Part model, mm, in its own coordinate system. A direction names the side the tool comes from. Round coordinates to 2 decimals unless told otherwise and drop trailing zeros. Write each loop counter-clockwise with the first axis right and the second up, starting at its lowest first coordinate (ties: lowest second). Pieces come first, ordered by that corner, then holes.
```python
from build123d import *

# Parameters (mm, degrees)
EXTRUDE_1_DEPTH     = 10
FILLET_1_R          = 2
CUT_EXTRUDE_1_DEPTH = 11
CUT_EXTRUDE_2_DEPTH = 11


with BuildPart() as part:
    # 草图1 → 凸台-拉伸1 (new body)
    with BuildSketch(Plane.XY):
        Polygon((-26.953865184, 1.151568381), (-21.953865184, 1.151568381), (-21.953865184, 11.151568381), (11.796134816, 11.151568381), (11.796134816, 1.151568381), (16.796134816, 1.151568381), (16.796134816, 16.151568381), (-26.953865184, 16.151568381), align=None)
    extrude(amount=EXTRUDE_1_DEPTH)

    # 圆角1
    fillet_1_edges = [part.edges().sort_by_distance(p)[0] for p in [
        (-26.953865184, 16.151568381, 5),
        (16.796134816, 16.151568381, 5),
    ]]
    fillet(fillet_1_edges, radius=FILLET_1_R)

    # 草图2 → 切除-拉伸1 (cut, through all)
    with BuildSketch(Plane.XY.offset(10)):
        Polygon((-26.953865184, 1.151568381), (-21.953865184, 1.151568381), (-26.953865184, 5.718181818), align=None)
    extrude(amount=-CUT_EXTRUDE_1_DEPTH, mode=Mode.SUBTRACT)

    # 草图3 → 切除-拉伸2 (cut, through all)
    with BuildSketch(Plane.XY.offset(10)):
        Polygon((16.796134816, 5.718181818), (11.796134816, 1.151568381), (16.796134816, 1.151568381), align=None)
    extrude(amount=-CUT_EXTRUDE_2_DEPTH, mode=Mode.SUBTRACT)


solid = part.part
```
Q1. Cut at C-C on x = -1. Write the cut outline in (y, z).
Values follow:
outline: (11.15, 0) - (16.15, 0) - (16.15, 10) - (11.15, 10) - close
Q2. Which spindle directions (+Z, -Z, +X, -X, +Y, -Y) get a long thin tool onto all of the face, cutting with end or side? Do faces 4 (the flat face through (11.796, 6, 5)), 5 (the cylindrical face through (16.226, 15.55, 5.07)). Say none if no direction does.
Values follow:
face 4: +Z, -Z, -Y
face 5: +Z, -Z, +X, +Y
Q3. Wall check: L1, parallel to X at y = 9.25, z = 6; L2, parallel to Y at x = -9.5, z = 0.75; L3, parallel to X at y = 4.75, z = 2.25. Give the ranges that are in metal, low to high.
Values follow:
L1: x = -26.95 to -21.95, 11.8 to 16.8
L2: y = 11.15 to 16.15
L3: x = -25.89 to -21.95, 11.8 to 15.74
Q4. Drop flat-ended pins along their axis: pin 1 (3 mm diameter, centred on x = 6, z = 5.5, fed in from -Y); pin 2 (4 mm diameter, centred on x = -21, y = 10, fed in from -Z). Give the stop position or say it passes through.
Values follow:
pin 1: stops at y = 11.15
pin 2: stops at z = 0
Q5. Cut at A-A on y = 9.5. Write the cut outline in (x, z).
Values follow:
outline: (-26.95, 0) - (-21.95, 0) - (-21.95, 10) - (-26.95, 10) - close; (11.8, 0) - (16.8, 0) - (16.8, 10) - (11.8, 10) - close
Q6. Cut at B-B on z = 9.25. Write the cut outline in (x, y).
Values follow:
outline: (-26.95, 5.72) - (-21.95, 1.15) - (-21.95, 11.15) - (11.8, 11.15) - (11.8, 1.15) - (16.8, 5.72) - (16.8, 14.15) arc R2 ccw to (14.8, 16.15) - (-24.95, 16.15) arc R2 ccw to (-26.95, 14.15) - close
Q7. Mould opens along X. For faces 1 (the flat face through (14.331, 3.467, 5.07)), 2 (the flat face through (-5, 11.152, 5)), 3 (the flat face through (-5, 12, 10)) say: +X half, -X half, draft (parallel to the pull), parting line (faces both ways), or undercut.
Values follow:
face 1: +X half
face 2: undercut
face 3: draft
Q8. Cut at D-D on x = -22.5. Write the cut outline in (y, z).
Values follow:
outline: (1.65, 0) - (16.15, 0) - (16.15, 10) - (1.65, 10) - close
